from build123d import *

# Parameters (mm, degrees)
F0_R     = 3
F0_R_2   = 1.075
F0_R_3   = 1.75
F1_DEPTH = 1.54
F2_R     = 6
F2_R_2   = 3.26
F3_DEPTH = 2.5


with BuildPart() as f1:
    # F0 (on Top) → F1 (new body)
    with BuildSketch(Plane.XY):
        with BuildLine():
            Line((28.115864, 4.065864), (4.065864, 28.115864))
            ThreePointArc((4.065864, 28.115864), (0, 29.8), (-4.065864, 28.115864))
            Line((-4.065864, 28.115864), (-28.115864, 4.065864))
            ThreePointArc((-28.115864, 4.065864), (-29.8, 0), (-28.115864, -4.065864))
            Line((-28.115864, -4.065864), (-4.065864, -28.115864))
            ThreePointArc((-4.065864, -28.115864), (0, -29.8), (4.065864, -28.115864))
            Line((4.065864, -28.115864), (28.115864, -4.065864))
            ThreePointArc((28.115864, -4.065864), (29.8, 0), (28.115864, 4.065864))
        make_face()
        with Locations((-24.05, 0)):
            Circle(F0_R, mode=Mode.SUBTRACT)
        with Locations((-12, 0)):
            Circle(F0_R_2, mode=Mode.SUBTRACT)
        with Locations((0, -24.05)):
            Circle(F0_R, mode=Mode.SUBTRACT)
        Circle(F0_R_3, mode=Mode.SUBTRACT)
        with Locations((12, 0)):
            Circle(F0_R_2, mode=Mode.SUBTRACT)
        with Locations((24.05, 0)):
            Circle(F0_R, mode=Mode.SUBTRACT)
        with Locations((0, 24.05)):
            Circle(F0_R, mode=Mode.SUBTRACT)
    extrude(amount=F1_DEPTH)

    # F2 (on face) → F3 (join)
    with BuildSketch(Plane.XY.offset(1.54)):
        Circle(F2_R)
        Circle(F2_R_2, mode=Mode.SUBTRACT)
    extrude(amount=F3_DEPTH)


solid = f1.part
Work out the finished part from the listing and answer in its coordinate system (mm). A direction names the side the tool comes from. Round coordinates to 2 decimals unless told otherwise and drop trailing zeros. Loops run counter-clockwise (first coordinate to the right, second up) from the corner with the lowest first, then second, coordinate; pieces in that order, holes last. Notation, with made-up numbers: (84, 21) -> (107, 21) arc R11 cw to (107, 28) -> close; hole circle Ø8 at (88, 68.25). An arc over 180 degrees is marked (long way). Use one line per item in the form item = value.
(1) Straight lines are drawn through the part: line 1 (Y direction, x = 0, z = 0.7); line 2 (Y direction, x = 0, z = 3.3); line 3 (Z direction, x = -3.5, y = 21.5). For each, find the intervals that lie inside material, in ascending order.
Answer list:
line_1 = -29.8 to -27.05, -21.05 to -1.75, 1.75 to 21.05, 27.05 to 29.8
line_2 = -6 to -3.26, 3.26 to 6
line_3 = 0 to 1.54
(2) A tool of negligible diameter and unlimited length cuts with its end or side. For faces 1 (the flat face through (1.4, -1.4, 1.54)), 2 (the cylindrical face through (-29.8, 0.1, 0.8)), from which of +Z, -Z, +X, -X, +Y, -Y can it reach the whole face along a straight path? Write none if from no direction.
Answer list:
face_1 = +Z
face_2 = +Z, -Z, -X
(3) For a pull along X with two mould halves and no side action, classify faces 3 (the flat face through (3, -3, 4.04)), 4 (the cylindrical face through (1.75, 2.75, 2.77)), 5 (the cylindrical face through (1.617, -0.67, 0.759)), 6 (the cylindrical face through (-0.1, -29.8, 0.8)) as released by +X, released by -X, zero draft, split by the parting line, or undercut.
Answer list:
face_3 = zero draft
face_4 = undercut
face_5 = undercut
face_6 = split by the parting line
(4) Find section A-A on y = 0. Give the number of separate pieces and of enclosed holes in the cut face, then the cut area to 3 significant figures.
Answer list:
separate_pieces = 6
enclosed_holes = 0
area = 75.0 mm2
(5) Find section B-B on x = -12. Give the vertices of the cut face in (y, z) (3 decimals).
Answer list:
outline = (-20.182, 0) -> (-1.075, 0) -> (-1.075, 1.54) -> (-20.182, 1.54) -> close; (1.075, 0) -> (20.182, 0) -> (20.182, 1.54) -> (1.075, 1.54) -> close
(6) Find section D-D on z = 3.2. Give the vertices of the cut face in (x, y), then the cut area to 3 significant figures.
Answer list:
outline = circle Ø12 at (0, 0); hole circle Ø6.52 at (0, 0)
area = 79.7 mm2
(7) Find section C-C on y = -22. Give the vertices of the cut face in (x, z), then the cut area to 3 significant figures.
Answer list:
outline = (-10.18, 0) -> (-2.19, 0) -> (-2.19, 1.54) -> (-10.18, 1.54) -> close; (2.19, 0) -> (10.18, 0) -> (10.18, 1.54) -> (2.19, 1.54) -> close
area = 24.6 mm2
(8) Flat-ended cylindrical pins translate along their axes: P1, Ø2.5, axis at x = 12, y = 0, coming from the +Z side; P2, Ø3, axis at x = 0, y = 0, coming from the +Z side; P3, Ø2, axis at y = 19, z = 2, coming from the -X side; P4, Ø1, axis at y = -2.5, z = 1, coming from the -X side. Find the tip coordinate at first contact, or state that the pin passes through.
Answer list:
P1 = 1.54
P2 = through
P3 = -14.07
P4 = -29.44
